```python
from build123d import *

# Parameters (mm, degrees)
BOSS_EXTRUDE1_DEPTH          = 3.175
F_10_0_1935_DIAMETER_HOLE1_D = 4.9149
F_1_4_CLEARANCE_HOLE2_D      = 6.7564
FILLET1_R                    = 7.62


with BuildPart() as part:
    # Sketch1 → Boss-Extrude1 (new body)
    with BuildSketch(Plane.XY):
        Polygon((0, 0), (82.55, 0), (82.55, 95.25), (165.1, 95.25), (165.1, 133.35), (44.45, 133.35), (44.45, 38.1), (0, 38.1), align=None)
    extrude(amount=BOSS_EXTRUDE1_DEPTH)

    # #10 (0.1935) Diameter Hole1 (through all)
    with Locations(Plane.XY.offset(3.175)):
        with Locations((63.5, 85.725), (63.5, 57.15), (63.5, 114.3), (149.225, 114.3), (104.775, 114.3)):
            Hole(F_10_0_1935_DIAMETER_HOLE1_D / 2)

    # 1/4 Clearance Hole2 (through all)
    with Locations(Plane.XY.offset(3.175)):
        with Locations((12.7, 19.05), (63.5, 19.05)):
            Hole(F_1_4_CLEARANCE_HOLE2_D / 2)

    # Fillet1
    fillet1_edges = [part.edges().sort_by_distance(p)[0] for p in [
        (0, 38.1, 1.5875),
        (44.45, 38.1, 1.5875),
        (44.45, 133.35, 1.5875),
        (165.1, 133.35, 1.5875),
        (165.1, 95.25, 1.5875),
        (82.55, 95.25, 1.5875),
        (82.55, 0, 1.5875),
        (0, 0, 1.5875),
    ]]
    fillet(fillet1_edges, radius=FILLET1_R)


solid = part.part
```
Could you check a few things on this model? Use its own coordinates, in mm. Round coordinates to 2 decimals unless told otherwise and drop trailing zeros. Loops run counter-clockwise (first coordinate to the right, second up) from the corner with the lowest first, then second, coordinate; pieces in that order, holes last. Notation, with made-up numbers: (7.5, -3.75) - (41.5, -3.75) arc R12 cw to (41.5, 19.25) - close; hole circle Ø8 at (-9.5, 69.5). An arc over 180 degrees is marked (long way). Answer in a Markdown table with one row per item. Add a question column.
(1) I'm going to push flat-ended pins straight in: pin 1 (3 mm diameter, centred on x = 149.225, y = 114.3, fed in from +Z); pin 2 (5 mm diameter, centred on x = 46, y = 33, fed in from -Z); pin 3 (1 mm diameter, centred on x = 19.5, z = 2, fed in from +Y); pin 4 (1 mm diameter, centred on y = 91, z = 1.5, fed in from -X). Where does each tip first touch, or does it pass through?
(2) If we mould it in two halves opening along X, with no side actions, what happens to faces 1 (the face through (2.173, 35.809, 1.61)), 2 (the face through (63.82, 88.16, 1.57)), 3 (the face through (13.43, 15.75, 1.57)), 4 (the face through (80.259, 2.173, 1.61))? For each: pulls with the +X half, pulls with the -X half, needs draft (parallel to the pull), parting line crosses it, or undercut.
(3) If we section it at C-C (x = 12.7): Please give me the cut outline in (y, z) (3 decimals), plus the area to 3 significant figures.
(4) I need wall thicknesses on line 1 along Y through (x, z) = (63.5, 1.1); line 2 along Y through (x, z) = (12.7, 1.6); line 3 along Y through (x, z) = (100.5, 2.1). Which ranges of each line are inside material? Lowest first, please.
(5) If we section it at A-A (x = 63.5): Please give me the cut outline in (y, z) (3 decimals).
(6) If we section it at B-B (y = 19.05): Please give me the cut outline in (x, z) (3 decimals), plus the area to 3 significant figures.
(7) If we section it at D-D (y = 114.3): Please give me the cut outline in (x, z) (3 decimals), plus the area to 3 significant figures.
Model answer:
| question | item | result |
|---|---|---|
| 1 | pin 1 | passes through |
| 1 | pin 2 | stops at z = 0 |
| 1 | pin 3 | stops at y = 38.1 |
| 1 | pin 4 | stops at x = 44.45 |
| 2 | face 1 | pulls with the -X half |
| 2 | face 2 | undercut |
| 2 | face 3 | undercut |
| 2 | face 4 | pulls with the +X half |
| 3 | outline | (0, 0) - (15.672, 0) - (15.672, 3.175) - (0, 3.175) - close; (22.428, 0) - (38.1, 0) - (38.1, 3.175) - (22.428, 3.175) - close |
| 3 | area | 99.5 mm² |
| 4 | line 1 | y = 0 to 15.67, 22.43 to 54.69, 59.61 to 83.27, 88.18 to 111.84, 116.76 to 133.35 |
| 4 | line 2 | y = 0 to 15.67, 22.43 to 38.1 |
| 4 | line 3 | y = 95.25 to 133.35 |
| 5 | outline | (0, 0) - (15.672, 0) - (15.672, 3.175) - (0, 3.175) - close; (22.428, 0) - (54.693, 0) - (54.693, 3.175) - (22.428, 3.175) - close; (59.607, 0) - (83.268, 0) - (83.268, 3.175) - (59.607, 3.175) - close; (88.182, 0) - (111.843, 0) - (111.843, 3.175) - (88.182, 3.175) - close; (116.757, 0) - (133.35, 0) - (133.35, 3.175) - (116.757, 3.175) - close |
| 6 | outline | (0, 0) - (9.322, 0) - (9.322, 3.175) - (0, 3.175) - close; (16.078, 0) - (60.122, 0) - (60.122, 3.175) - (16.078, 3.175) - close; (66.878, 0) - (82.55, 0) - (82.55, 3.175) - (66.878, 3.175) - close |
| 6 | area | 219 mm² |
| 7 | outline | (44.45, 0) - (61.043, 0) - (61.043, 3.175) - (44.45, 3.175) - close; (65.957, 0) - (102.318, 0) - (102.318, 3.175) - (65.957, 3.175) - close; (107.232, 0) - (146.768, 0) - (146.768, 3.175) - (107.232, 3.175) - close; (151.682, 0) - (165.1, 0) - (165.1, 3.175) - (151.682, 3.175) - close |
| 7 | area | 336 mm² |
